Model file for the job. Use its own axes, mm. A direction names the side the tool comes from. Coordinates: 2 decimals unless noted, no trailing zeros. Loops run counter-clockwise (first coordinate to the right, second up) from the corner with the lowest first, then second, coordinate; pieces in that order, holes last. Notation, with made-up numbers: (-21, -16) -> (14, -16) arc R17 ccw to (14, -7) -> close; hole circle Ø3 at (89.25, 66.25). An arc over 180 degrees is marked (long way). Use one line per item in the form item = value.
```python
from build123d import *

# Parameters (mm, degrees)
SKETCH2_R           = 1.65
CUT_EXTRUDE1_DEPTH  = 20
SKETCH3_W           = 1
SKETCH3_H           = 5
BOSS_EXTRUDE1_DEPTH = 8


with BuildPart() as part:
    # Sketch1 → Revolve1 (revolve)
    with BuildSketch(Plane.XY):
        Polygon((0, 0), (0, 105), (2.5, 105), (2.5, 89), (8.75, 89), (8.75, 84), (21, 84), (21, 79), (22.5, 79), (22.5, 44), (21, 44), (21, 8), (8.75, 8), (8.75, 3), (2.5, 3), (2.5, 0), align=None)
    revolve(axis=Axis((0, 0, 0), (0, 1, 0)))

    # Sketch2 → Cut-Extrude1 (cut)
    with BuildSketch(Plane(origin=(0, 84, 0), x_dir=(1, 0, 0), z_dir=(0, 1, 0))):
        with Locations((14.5, 0)):
            Circle(SKETCH2_R)
        with Locations((-14.5, 0)):
            Circle(SKETCH2_R)
    extrude(amount=-CUT_EXTRUDE1_DEPTH, mode=Mode.SUBTRACT)

    # Sketch3 → Boss-Extrude1 (add)
    with BuildSketch(Plane.XZ.offset(-8)):
        with Locations((-18, 0)):
            Rectangle(SKETCH3_W, SKETCH3_H)
        with Locations((18, 0)):
            Rectangle(SKETCH3_W, SKETCH3_H)
    extrude(amount=BOSS_EXTRUDE1_DEPTH)


solid = part.part
```
Q1. Band-saw the part on C-C, the plane z = 7.5. Write the cut outline in (x, y), and give its area (3 significant figures).
Result:
outline = (-21.21, 44) -> (-19.62, 44) -> (-19.62, 8) -> (-4.51, 8) -> (-4.51, 3) -> (4.51, 3) -> (4.51, 8) -> (19.62, 8) -> (19.62, 44) -> (21.21, 44) -> (21.21, 79) -> (19.62, 79) -> (19.62, 84) -> (4.51, 84) -> (4.51, 89) -> (-4.51, 89) -> (-4.51, 84) -> (-19.62, 84) -> (-19.62, 79) -> (-21.21, 79) -> close
area = 3,180 mm2
Q2. Band-saw the part on A-A, the plane y = 73.5. Write the cut outline in (x, z), and give its area (3 significant figures).
Result:
outline = circle Ø45 at (0, 0); hole circle Ø3.3 at (-14.5, 0); hole circle Ø3.3 at (14.5, 0)
area = 1,570 mm2
Q3. Pin check, flat tips, straight feed: pin 1 Ø8 at (x, y) = (-17.5, 37) entering from +Z; pin 2 Ø2 at (y, z) = (76.5, -16.5) entering from -X; pin 3 Ø4 at (y, z) = (3.5, 1) entering from -X. Stop position of each tip, or through.
Result:
pin_1 = 16.09
pin_2 = -16.31
pin_3 = -18.5
Q4. Mould opens along Z. For faces 1 (the face through (-17.5, 4, 0)), 2 (the face through (14, 64, 0)), 3 (the face through (20.03, 25.75, -6.31)) say: released by +Z, released by -Z, zero draft, split by the parting line, or undercut.
Result:
face_1 = zero draft
face_2 = undercut
face_3 = split by the parting line
Q5. Wall check: line 1 along X through (y, z) = (70, 0); line 2 along Y through (x, z) = (-9, -1.5); line 3 along Y through (x, z) = (18, -0.5). Give the ranges that are in metal, low to high.
Result:
line_1 = -22.5 to -16.15, -12.85 to 12.85, 16.15 to 22.5
line_2 = 8 to 84
line_3 = 0 to 84
Q6. Which spindle directions (+Z, -Z, +X, -X, +Y, -Y) get a long thin tool onto all of the face, cutting with end or side? Do faces 4 (the face through (-6.944, 5.465, 5.324)), 5 (the face through (-18.5, 4, 0)), 6 (the face through (17.5, 4, 0)), 7 (the face through (0, 0, 0)), 8 (the face through (-15, 64, 0)). Say none if no direction does.
Result:
face_4 = -Y
face_5 = +Z, -Z, -X, -Y
face_6 = +Z, -Z, -Y
face_7 = +Z, -Z, +X, -X, -Y
face_8 = +Y
Q7. Band-saw the part on B-B, the plane x = 0. Write the cut outline in (y, z).
Result:
outline = (0, -2.5) -> (3, -2.5) -> (3, -8.75) -> (8, -8.75) -> (8, -21) -> (44, -21) -> (44, -22.5) -> (79, -22.5) -> (79, -21) -> (84, -21) -> (84, -8.75) -> (89, -8.75) -> (89, -2.5) -> (105, -2.5) -> (105, 2.5) -> (89, 2.5) -> (89, 8.75) -> (84, 8.75) -> (84, 21) -> (79, 21) -> (79, 22.5) -> (44, 22.5) -> (44, 21) -> (8, 21) -> (8, 8.75) -> (3, 8.75) -> (3, 2.5) -> (0, 2.5) -> close
Q8. Band-saw the part on D-D, the plane y = 88. Write the cut outline in (x, z), and give its area (3 significant figures).
Result:
outline = circle Ø17.5 at (0, 0)
area = 241 mm2
